```python
from build123d import *

# Parameters (mm, degrees)
ESQUISSE1_W             = 50
ESQUISSE1_H             = 42
ESQUISSE1_R             = 1.75
BOSS_EXTRU_1_DEPTH      = 4
ESQUISSE2_W             = 6
ESQUISSE2_H             = 5
BOSS_EXTRU_2_DEPTH      = 35.5
ESQUISSE3_R             = 1.25
ENL_V_MAT_EXTRU_1_DEPTH = 43
CONG_1_R                = 2


with BuildPart() as part:
    # Esquisse1 → Boss.-Extru.1 (new body)
    with BuildSketch(Plane.XY):
        Rectangle(ESQUISSE1_W, ESQUISSE1_H)
        with Locations((-19, 11)):
            Circle(ESQUISSE1_R, mode=Mode.SUBTRACT)
        with Locations((19, 11)):
            Circle(ESQUISSE1_R, mode=Mode.SUBTRACT)
        with Locations((19, -11)):
            Circle(ESQUISSE1_R, mode=Mode.SUBTRACT)
        with Locations((-19, -11)):
            Circle(ESQUISSE1_R, mode=Mode.SUBTRACT)
    extrude(amount=BOSS_EXTRU_1_DEPTH)

    # Esquisse2 → Boss.-Extru.2 (add)
    with BuildSketch(Plane.XY.offset(4)):
        with Locations((-13.5, 18.5)):
            Rectangle(ESQUISSE2_W, ESQUISSE2_H)
        with Locations((13.5, 18.5)):
            Rectangle(ESQUISSE2_W, ESQUISSE2_H)
        with Locations((-13.5, -18.5)):
            Rectangle(ESQUISSE2_W, ESQUISSE2_H)
        with Locations((13.5, -18.5)):
            Rectangle(ESQUISSE2_W, ESQUISSE2_H)
    extrude(amount=BOSS_EXTRU_2_DEPTH)

    # Esquisse3 → Enlèv. mat.-Extru.1 (cut, through all)
    with BuildSketch(Plane(origin=(0, 21, 0), x_dir=(1, 0, 0), z_dir=(0, 1, 0))):
        with Locations((-13.5, -12)):
            Circle(ESQUISSE3_R)
        with Locations((-13.5, -20)):
            Circle(ESQUISSE3_R)
        with Locations((-13.5, -28)):
            Circle(ESQUISSE3_R)
        with Locations((-13.5, -36)):
            Circle(ESQUISSE3_R)
        with Locations((13.5, -36)):
            Circle(ESQUISSE3_R)
        with Locations((13.5, -28)):
            Circle(ESQUISSE3_R)
        with Locations((13.5, -20)):
            Circle(ESQUISSE3_R)
        with Locations((13.5, -12)):
            Circle(ESQUISSE3_R)
    extrude(amount=-ENL_V_MAT_EXTRU_1_DEPTH, mode=Mode.SUBTRACT)

    # Congé1
    cong_1_edges = [part.edges().sort_by_distance(p)[0] for p in [
        (-16.5, 18.5, 4),
        (-10.5, 18.5, 4),
        (-16.5, 18.5, 39.5),
        (-10.5, 18.5, 39.5),
        (16.5, 18.5, 4),
        (10.5, 18.5, 4),
        (16.5, 18.5, 39.5),
        (10.5, 18.5, 39.5),
        (-10.5, -18.5, 4),
        (-16.5, -18.5, 4),
        (-10.5, -18.5, 39.5),
        (-16.5, -18.5, 39.5),
        (16.5, -18.5, 4),
        (10.5, -18.5, 4),
        (16.5, -18.5, 39.5),
        (10.5, -18.5, 39.5),
    ]]
    fillet(cong_1_edges, radius=CONG_1_R)


solid = part.part
```
Geometry: final body of the model. Coordinates: model frame, mm. A direction names the side the tool comes from. Coordinates: 2 decimals unless noted, no trailing zeros. Loops run counter-clockwise (first coordinate to the right, second up) from the corner with the lowest first, then second, coordinate; pieces in that order, holes last. Notation, with made-up numbers: (9.5, -38.75) -> (16.5, -38.75) arc R23 ccw to (16.5, -28.75) -> close; hole circle Ø11 at (30.5, 68). An arc over 180 degrees is marked (long way). Use a Markdown table: item, result. Add a question column.
(1) Line query: line 1 along Y through (x, z) = (19, 1.15); line 2 along X through (y, z) = (-19, 36); line 3 along Y through (x, z) = (12, 15.5). Output: solid intervals per line, ascending.
(2) Access query for faces 4 (the flat face through (13, -16, 22)), 5 (the cylindrical face through (17.1, -18.46, 4.57)), 6 (the cylindrical face through (11.1, -18.46, 38.93)). Directions: +Z, -Z, +X, -X, +Y, -Y. A direction counts if a zero-diameter tool reaches every point of the face in a straight line with its end or side. Return the directions, or none.
(3) Mould query, pull axis Z, two halves, no side actions, for faces 1 (the cylindrical face through (-13.77, -18.47, 37.22)), 2 (the flat face through (-14, 19, 39.5)), 3 (the flat face through (-25, 0, 2)). Classes: pulls with the +Z half, pulls with the -Z half, needs draft (parallel to the pull), parting line crosses it, or undercut.
(4) Section query A-A, the plane z = 28. State how many separate pieces and enclosed holes the cut face has, plus the area to 3 significant figures.
(5) Pin query (flat end, axial travel): pin 1 Ø3 at (x, y) = (6, 6.5) entering from +Z; pin 2 Ø3 at (y, z) = (-16.5, 14) entering from +X; pin 3 Ø12 at (x, z) = (5.5, 35) entering from +Y; pin 4 Ø4 at (y, z) = (-19.5, 17) entering from -X. Return the tip coordinate at first contact, or that it passes through.
(6) Section query B-B, the plane y = -11. Return loops of the section in (x, z).
(7) Section query D-D, the plane z = 23.5. Return loops of the section in (x, y).
Answer:
| question | item | result |
|---|---|---|
| 1 | line 1 | y = -21 to -12.75, -9.25 to 9.25, 12.75 to 21 |
| 1 | line 2 | x = -16.5 to -14.75, -12.25 to -10.5, 10.5 to 12.25, 14.75 to 16.5 |
| 1 | line 3 | y = -21 to -16, 16 to 21 |
| 2 | face 4 | +Z, +X, -X |
| 2 | face 5 | +Z, +X, +Y, -Y |
| 2 | face 6 | +Z, +Y, -Y |
| 3 | face 1 | undercut |
| 3 | face 2 | pulls with the +Z half |
| 3 | face 3 | needs draft |
| 4 | separate pieces | 8 |
| 4 | enclosed holes | 0 |
| 4 | area | 70.0 mm^2 |
| 5 | pin 1 | stops at z = 4 |
| 5 | pin 2 | stops at x = 16.5 |
| 5 | pin 3 | stops at y = 21 |
| 5 | pin 4 | stops at x = -16.5 |
| 6 | outline | (-25, 0) -> (-20.75, 0) -> (-20.75, 4) -> (-25, 4) -> close; (-17.25, 0) -> (17.25, 0) -> (17.25, 4) -> (-17.25, 4) -> close; (20.75, 0) -> (25, 0) -> (25, 4) -> (20.75, 4) -> close |
| 7 | outline | (-16.5, -21) -> (-10.5, -21) -> (-10.5, -16) -> (-16.5, -16) -> close; (-16.5, 16) -> (-10.5, 16) -> (-10.5, 21) -> (-16.5, 21) -> close; (10.5, -21) -> (16.5, -21) -> (16.5, -16) -> (10.5, -16) -> close; (10.5, 16) -> (16.5, 16) -> (16.5, 21) -> (10.5, 21) -> close |
